Work out the finished part from the listing and answer in its coordinate system (mm). Coordinates: 2 decimals unless noted, no trailing zeros. Loops run counter-clockwise (first coordinate to the right, second up) from the corner with the lowest first, then second, coordinate; pieces in that order, holes last. Notation, with made-up numbers: (23.5, 41) - (70.5, 41) arc R25 ccw to (70.5, 68) - close; hole circle Ø6 at (-2.5, 59). An arc over 180 degrees is marked (long way). Write each question's results on one line, items separated by ' | '. Start each with the question number.
Item 1: Consider probe 1 along Z at (x, y) = (19, 3); probe 2 along Y at (x, z) = (23, 17.5); probe 3 along Y at (x, z) = (11, 8.5). Determine where each line is inside the solid, lowest interval first. Write a range as [from, to].
Item 2: Section B-B, the plane x = 0 is taken. Write down the section's boundary in (y, z), plus the area to 3 significant figures.
Item 3: Section C-C, the plane y = 19 is taken. Write down the section's boundary in (x, z).
Item 4: Section A-A, the plane z = 0 is taken. Write down the section's boundary in (x, y), plus the area to 3 significant figures.
Item 5: For a pull along X with two mould halves and no side action, classify faces 1 (the face through (12.4, 2.75, -22.68)), 2 (the face through (-6.8, 5.588, -12.5)), 3 (the face through (19.89, 2.75, 12.32)), 4 (the face through (-6.324, 14.65, -4.032)) as +X half, -X half, draft (parallel to the pull), parting line (faces both ways), or undercut.
Item 6: Section D-D, the plane y = 24.5 is taken. Write down the section's boundary in (x, z).
Item 7: Each of these flat-tipped pins is pushed along its axis until it touches: pin 1 Ø6 at (y, z) = (46.5, -13.5) entering from +X; pin 2 Ø8 at (y, z) = (33, -12.5) entering from -X; pin 3 Ø5 at (x, y) = (13.5, 40.5) entering from +Z. Where does it stop, or does it pass through?
from build123d import *

# Parameters (mm, degrees)
SKETCH2_R          = 2.794
CUT_EXTRUDE1_DEPTH = 10


with BuildPart() as part:
    # Sketch1 → Revolve1 (revolve)
    with BuildSketch(Plane.XY, mode=Mode.PRIVATE) as revolve1_sk:
        with BuildLine():
            Line((0, 0), (30.988, 0))
            Line((30.988, 0), (30.988, 3.588))
            ThreePointArc((30.988, 3.588), (30.402213562, 5.002213562), (28.988, 5.588))
            Line((28.988, 5.588), (13.85, 5.588))
            ThreePointArc((13.85, 5.588), (9.359871939, 7.447871939), (7.5, 11.938))
            Line((7.5, 11.938), (7.5, 17.286503776))
            ThreePointArc((7.5, 17.286503776), (18.661410759, 38.626086789), (0, 53.848))
            Line((0, 53.848), (0, 0))
        make_face()
    revolve(revolve1_sk.sketch.rotate(Axis((0, 0, 0), (0, 1, 0)), 90), axis=Axis((0, 0, 0), (0, 1, 0)))

    # Sketch2 → Cut-Extrude1 (cut)
    with BuildSketch(Plane.XZ):
        with Locations(Location((-23.114, 0, 0), (0, 0, 270))):
            Circle(SKETCH2_R)
        with Locations(Location((11.557, 20.017311183, 0), (0, 0, 270))):
            Circle(SKETCH2_R)
        with Locations(Location((11.557, -20.017311183, 0), (0, 0, 270))):
            Circle(SKETCH2_R)
        with Locations(Location((-19.05, 14.986, 0), (0, 0, 270))):
            Circle(SKETCH2_R)
        with Locations(Location((19.05, 14.986, 0), (0, 0, 270))):
            Circle(SKETCH2_R)
        with Locations(Location((19.05, -14.986, 0), (0, 0, 270))):
            Circle(SKETCH2_R)
        with Locations(Location((-19.05, -14.986, 0), (0, 0, 270))):
            Circle(SKETCH2_R)
    extrude(amount=-CUT_EXTRUDE1_DEPTH, mode=Mode.SUBTRACT)


solid = part.part
Answer key:
1) probe 1: z = [-24.48, -17.78], [-12.19, 12.19], [17.78, 24.48] | probe 2: y = [0, 5.59] | probe 3: y = [0, 5.59], [21.77, 47.82]
2) outline: (0, -30.99) - (3.59, -30.99) arc R2 ccw to (5.59, -28.99) - (5.59, -13.85) arc R6.35 cw to (11.94, -7.5) - (17.29, -7.5) arc R19.05 ccw (long way) to (17.29, 7.5) - (11.94, 7.5) arc R6.35 cw to (5.59, 13.85) - (5.59, 28.99) arc R2 ccw to (3.59, 30.99) - (0, 30.99) - close | area: 1,660 mm^2
3) outline: circle Ø21.29 at (0, 0)
4) outline: (-30.99, 0) - (-25.91, 0) - (-25.91, 5.59) - (-28.99, 5.59) arc R2 ccw to (-30.99, 3.59) - close; (-20.32, 0) - (30.99, 0) - (30.99, 3.59) arc R2 ccw to (28.99, 5.59) - (13.85, 5.59) arc R6.35 cw to (7.5, 11.94) - (7.5, 17.29) arc R19.05 ccw (long way) to (-7.5, 17.29) - (-7.5, 11.94) arc R6.35 cw to (-13.85, 5.59) - (-20.32, 5.59) - close | area: 1,630 mm^2
5) face 1: undercut | face 2: draft | face 3: undercut | face 4: parting line
6) outline: circle Ø32.05 at (0, 0)
7) pin 1: stops at x = 11.91 | pin 2: stops at x = -16.98 | pin 3: stops at z = 14.67
